Can you work these out from the model? Positions are in its coordinate system, mm. A direction names the side the tool comes from. Coordinates: 2 decimals unless noted, no trailing zeros. Order: outer loops, then holes, each group sorted by start corner. A loop starts at its lowest first (then second) coordinate and runs counter-clockwise, first axis right, second up. Notation, with made-up numbers: M 64.25,6 L 98.25,6 A20 ccw 98.25,16 Z; hole C -8.5,-18.5 d10. An arc over 180 degrees is marked long. Answer as a JSON object with one key per item and string values.
from build123d import *

# Parameters (mm, degrees)
BOSS_EXTRUDE2_DEPTH      = 10
BOSS_EXTRUDE2_DEPTH_BACK = 10
EXTRUDE_THIN2_START      = -10
EXTRUDE_THIN2_DEPTH      = 20
SKETCH2_W                = 20
SKETCH2_H                = 2.5
BOSS_EXTRUDE3_DEPTH      = 90


# Read off the part's stored shape, not the designer's step: Extrude-Thin2
with BuildPart() as part:
    # Sketch1 → Boss-Extrude2 (new, two sides: drawn at the far end of the back side and taken through both)
    with BuildSketch(Plane.XY.offset(-BOSS_EXTRUDE2_DEPTH_BACK)):
        Polygon((-13.01396445, -23.830717844), (0, -23.830717844), (0, -18.830717844), (-11.698214449, -18.830717844), (-45, 0), (-45, 13.432214294), (-50, 13.432214294), (-50, -2.916716145), align=None)
        Polygon((0, -18.830717844), (0, -23.830717844), (13.01396445, -23.830717844), (50, -2.916716145), (50, 13.432214294), (45, 13.432214294), (45, 0), (11.698214449, -18.830717844), align=None)
        with BuildLine():
            Line((-11.698214449, -18.830717844), (0, -18.830717844))
            Line((0, -18.830717844), (0, -8))
            ThreePointArc((0, -8), (-8, 0), (0, 8))
            Line((0, 8), (0, 13.432214294))
            Line((0, 13.432214294), (-45, 13.432214294))
            Line((-45, 13.432214294), (-45, 0))
            Line((-45, 0), (-11.698214449, -18.830717844))
        make_face()
        with BuildLine():
            Line((0, -8), (0, -18.830717844))
            Line((0, -18.830717844), (11.698214449, -18.830717844))
            Line((11.698214449, -18.830717844), (45, 0))
            Line((45, 0), (45, 13.432214294))
            Line((45, 13.432214294), (0, 13.432214294))
            Line((0, 13.432214294), (0, 8))
            ThreePointArc((0, 8), (5.656854249, 5.656854249), (8, 0))
            ThreePointArc((8, 0), (5.656854249, -5.656854249), (0, -8))
        make_face()
    extrude(amount=BOSS_EXTRUDE2_DEPTH + BOSS_EXTRUDE2_DEPTH_BACK)

    # Extrude-Thin2 outline → Extrude-Thin2 (add)
    with BuildSketch(Plane.XY.offset(EXTRUDE_THIN2_START)):
        Polygon((45, 13.432214294), (50, 13.432214294), (50, 68.432214294), (-50, 68.432214294), (-50, 13.432214294), (-45, 13.432214294), (-45, 63.432214294), (45, 63.432214294), align=None)
    extrude(amount=EXTRUDE_THIN2_DEPTH)

    # Sketch2 → Boss-Extrude3 (add)
    with BuildSketch(Plane.ZY.offset(-45)):
        with Locations((0, 38.944873029)):
            Rectangle(SKETCH2_W, SKETCH2_H)
        with Locations((0, 36.444873029)):
            Rectangle(SKETCH2_W, SKETCH2_H)
    extrude(amount=BOSS_EXTRUDE3_DEPTH)


solid = part.part
Item 1: I want a section at D-D, the plane y = 4. Write out the boundary of the cut face in (x, z), plus the area to 3 significant figures.
Answers follow:
{"outline": "M -50,-10 L -6.93,-10 L -6.93,10 L -50,10 Z; M 6.93,-10 L 50,-10 L 50,10 L 6.93,10 Z", "area": "1,720 mm^2"}
Item 2: If we mould it in two halves opening along X, with no side actions, what happens to faces 1 (the flat face through (1, 40.195, 0)), 2 (the flat face through (50, 32, 0)), 3 (the flat face through (-1, 13, 10))? For each: pulls with the +X half, pulls with the -X half, needs draft (parallel to the pull), parting line crosses it, or undercut.
Answers follow:
{"face 1": "undercut", "face 2": "pulls with the +X half", "face 3": "needs draft"}
Item 3: I'm going to push flat-ended pins straight in: pin 1 (6 mm diameter, centred on x = -21, z = 2, fed in from -Y); pin 2 (5 mm diameter, centred on x = 21, z = -3, fed in from -Y); pin 3 (1 mm diameter, centred on x = 29, z = -1.5, fed in from -Y). Where does each tip first touch, or does it pass through?
Answers follow:
{"pin 1": "stops at y = -21.01", "pin 2": "stops at y = -20.73", "pin 3": "stops at y = -15.07"}
Item 4: I want a section at B-B, the plane z = 0.25. Write out the boundary of the cut face in (x, y), plus the area to 3 significant figures.
Answers follow:
{"outline": "M -50,-2.92 L -13.01,-23.83 L 13.01,-23.83 L 50,-2.92 L 50,68.43 L -50,68.43 Z; hole M -45,13.43 L 45,13.43 L 45,35.19 L -45,35.19 Z; hole M -45,40.19 L 45,40.19 L 45,63.43 L -45,63.43 Z; hole C 0,0 d16", "area": "4,200 mm^2"}
Item 5: I want a section at A-A, the plane y = 58. Write out the boundary of the cut face in (x, z), plus the area to 3 significant figures.
Answers follow:
{"outline": "M -50,-10 L -45,-10 L -45,10 L -50,10 Z; M 45,-10 L 50,-10 L 50,10 L 45,10 Z", "area": "200 mm^2"}
Item 6: Please list where these lines run through material, in increasing order: line 1 (Y direction, x = -11, z = 5); line 2 (X direction, y = 61.5, z = 8.5); line 3 (Y direction, x = -16.5, z = 7.25).
Answers follow:
{"line 1": "y = -23.83 to 13.43, 35.19 to 40.19, 63.43 to 68.43", "line 2": "x = -50 to -45, 45 to 50", "line 3": "y = -21.86 to 13.43, 35.19 to 40.19, 63.43 to 68.43"}
Item 7: I want a section at C-C, the plane x = 31.5. Write out the boundary of the cut face in (y, z), plus the area to 3 significant figures.
Answers follow:
{"outline": "M -13.38,-10 L 13.43,-10 L 13.43,10 L -13.38,10 Z; M 35.19,-10 L 40.19,-10 L 40.19,10 L 35.19,10 Z; M 63.43,-10 L 68.43,-10 L 68.43,10 L 63.43,10 Z", "area": "736 mm^2"}
Item 8: Which directions (+Z, -Z, +X, -X, +Y, -Y) give clear straight access to the entire face, cutting with the end or side of a thin tool? Please do faces 4 (the flat face through (-1, 63.432, 0)), 5 (the flat face through (0, -23.831, 0)).
Answers follow:
{"face 4": "+Z, -Z", "face 5": "+Z, -Z, +X, -X, -Y"}
